Autodesk Inventor part; units mm, degrees
ref_plane "YZ Plane" through (0, 0, 0) normal (1, 0, 0) x (0, 1, 0)
ref_plane "XZ Plane" through (0, 0, 0) normal (0, 1, 0) x (-1, 0, 0)
ref_plane "XY Plane" through (0, 0, 0) normal (0, 0, 1) x (1, 0, 0)
ref_plane "Work Plane1" through (-28.594, 4.5215, 39.249) normal (0, 0, 1) x (1, 0, 0)
sketch "Sketch1" plane through (-28.594, 4.5215, 39.249) normal (0, 0, 1) x (1, 0, 0)
  circle A0 centre (23.594, 21.5215) radius 1.45
  circle A1 centre (-23.594, 21.5215) radius 1.45
  circle A2 centre (23.594, 21.5215) radius 1.45
  arc A3 (-26.094, 26.5215) -> (-28.594, 24.0215) centre (-26.094, 24.0215) ccw
  line L0 (26.094, 26.5215) -> (-26.094, 26.5215)
  arc A4 (28.594, 24.0215) -> (26.094, 26.5215) centre (26.094, 24.0215) ccw
  line L1 (28.594, 19.0215) -> (28.594, 24.0215)
  arc A5 (26.094, 16.5215) -> (28.594, 19.0215) centre (26.094, 19.0215) ccw
  line L2 (-26.094, 16.5215) -> (26.094, 16.5215)
  arc A6 (-28.594, 19.0215) -> (-26.094, 16.5215) centre (-26.094, 19.0215) ccw
  line L3 (-28.594, 24.0215) -> (-28.594, 19.0215)
  circle A7 centre (-23.594, 21.5215) radius 1.45
  point P0 (28.594, -4.5215)
extrude "Extrusion1" add sketch "Sketch1" along normal blind 7.842
sketch "Sketch2" plane through (-54.688, 31.043, 39.249) normal (0, 1, 0) x (1, 0, 0)
  line L0 (32.3438, -5.842) -> (19.8438, -5.842) construction
  line L1 (19.8438, -5.842) -> (19.8438, 0) construction
  line L2 (19.8438, 0) -> (32.3438, 0) construction
  line L3 (32.3438, 0) -> (32.3438, -5.842) construction
  line L4 (52.188, 0) -> (0, 0)
  line L5 (32.4438, 0) -> (32.4438, -6.042)
  line L6 (32.4438, -6.042) -> (19.7438, -6.042)
  line L7 (19.7438, -6.042) -> (19.7438, 0)
  point P0 (54.688, 39.249)
  dimension "d2" = 0.1
  dimension "d3" = 0.1
  dimension "d4" = 0.2
extrude "Extrusion2" cut sketch "Sketch2" against normal blind 12.908
ref_plane "Work Plane2" through (-52.188, -17, 42.6) normal (0, 0, -1) x (0, 1, 0)
sketch "Sketch3" plane through (-52.188, -17, 42.6) normal (0, 0, -1) x (0, 1, 0)
  line L0 (45.543, -5) -> (40.543, -5)
  arc A0 (38.043, -2.5) -> (40.543, -5) centre (40.543, -2.5) ccw
  line L1 (38.043, -2.5) -> (38.043, 49.688)
  arc A1 (40.543, 52.188) -> (38.043, 49.688) centre (40.543, 49.688) ccw
  line L2 (40.543, 52.188) -> (45.543, 52.188)
  arc A2 (48.043, 49.688) -> (45.543, 52.188) centre (45.543, 49.688) ccw
  line L3 (48.043, 49.688) -> (48.043, -2.5)
  arc A3 (45.543, -5) -> (48.043, -2.5) centre (45.543, -2.5) ccw
  circle A4 centre (43.043, 47.188) radius 1.45
  circle A5 centre (43.043, 0) radius 1.45
  circle A6 centre (0, 47.188) radius 3.065
  circle A7 centre (43.043, 47.188) radius 3.065
  circle A8 centre (43.043, 0) radius 3.065
  point P0 (17, 52.188)
extrude "Extrusion3" cut sketch "Sketch3" against normal blind 12.908 contours A4 | A5 | A7 | A8
properties part number "connectorHolder_V6"
Could you check a few things on this model? Use its own coordinates, in mm. A direction names the side the tool comes from. Round coordinates to 2 decimals unless told otherwise and drop trailing zeros. Write each loop counter-clockwise with the first axis right and the second up, starting at its lowest first coordinate (ties: lowest second). Pieces come first, ordered by that corner, then holes. Notation, with made-up numbers: (-20.75, -34.5) -> (33.25, -34.5) arc R21 ccw to (33.25, 1.5) -> close; hole circle Ø8 at (25.25, 43.25). An arc over 180 degrees is marked (long way). Use a Markdown table: item, result.
1. Which directions (+Z, -Z, +X, -X, +Y, -Y) give clear straight access to the entire face, cutting with the end or side of a thin tool? Please do faces 5 (the face through (-22.244, 26, 42)), 6 (the face through (-11, 26, 39.249)), 7 (the face through (-6.174, 28.874, 44.814)).
Answer key:
| item | result |
|---|---|
| face 5 | -Z, +Y, -Y |
| face 6 | -Z, +X, -X, +Y, -Y |
| face 7 | +Z |
2. If we section it at D-D (z = 46.5): List the corners of the cut face in (x, y) for me (3 decimals).
Answer key:
| item | result |
|---|---|
| outline | (-57.188, 23.543) arc R2.5 ccw to (-54.688, 21.043) -> (-2.5, 21.043) arc R2.5 ccw to (0, 23.543) -> (0, 28.543) arc R2.5 ccw to (-2.5, 31.043) -> (-54.688, 31.043) arc R2.5 ccw to (-57.188, 28.543) -> close; hole circle Ø6.13 at (-52.188, 26.043); hole circle Ø6.13 at (-5, 26.043) |
3. Please list where these lines run through material, in increasing order: probe 1 along X at (y, z) = (28, 42.5); probe 2 along X at (y, z) = (25, 46); probe 3 along Y at (x, z) = (-5, 40.95).
Answer key:
| item | result |
|---|---|
| probe 1 | x = -57.19 to -34.94, -22.24 to 0 |
| probe 2 | x = -57.19 to -55.07, -49.31 to -7.88, -2.12 to 0 |
| probe 3 | y = 21.04 to 24.59, 27.49 to 31.04 |
4. If we section it at C-C (y = 26.75): List the corners of the cut face in (x, z) for me.
Answer key:
| item | result |
|---|---|
| outline | (-57.19, 39.25) -> (-53.45, 39.25) -> (-53.45, 42.6) -> (-55.17, 42.6) -> (-55.17, 47.09) -> (-57.19, 47.09) -> close; (-50.92, 39.25) -> (-34.94, 39.25) -> (-34.94, 45.29) -> (-22.24, 45.29) -> (-22.24, 39.25) -> (-6.27, 39.25) -> (-6.27, 42.6) -> (-7.98, 42.6) -> (-7.98, 47.09) -> (-49.21, 47.09) -> (-49.21, 42.6) -> (-50.92, 42.6) -> close; (-3.73, 39.25) -> (0, 39.25) -> (0, 47.09) -> (-2.02, 47.09) -> (-2.02, 42.6) -> (-3.73, 42.6) -> close |
5. If we section it at A-A (x = -5): List the corners of the cut face in (y, z) for me, then the cut area to 3 significant figures.
Answer key:
| item | result |
|---|---|
| outline | (21.04, 39.25) -> (24.59, 39.25) -> (24.59, 42.6) -> (22.98, 42.6) -> (22.98, 47.09) -> (21.04, 47.09) -> close; (27.49, 39.25) -> (31.04, 39.25) -> (31.04, 47.09) -> (29.11, 47.09) -> (29.11, 42.6) -> (27.49, 42.6) -> close |
| area | 41.2 mm^2 |
6. For pin 1 Ø5 at (x, y) = (-26.5, 28) entering from -Z; pin 2 Ø1.8 at (x, y) = (-53, 27.5) entering from +Z; pin 3 Ø1.5 at (y, z) = (22.5, 46) entering from -X, each with a flat end and sliding along its axis, tell me the tip position at first contact or that it passes through.
Answer key:
| item | result |
|---|---|
| pin 1 | stops at z = 45.29 |
| pin 2 | stops at z = 42.6 |
| pin 3 | stops at x = -57.17 |
7. We'd pull the mould along X, two halves only. Please class faces 1 (the face through (-0.713, 21.795, 43.115)), 2 (the face through (-56.44, 21.76, 43.12)), 3 (the face through (-34.944, 26, 42)), 4 (the face through (-51.267, 28.966, 44.814)): +X half, -X half, draft (parallel to the pull), parting line (faces both ways), or undercut.
Answer key:
| item | result |
|---|---|
| face 1 | +X half |
| face 2 | -X half |
| face 3 | undercut |
| face 4 | undercut |
8. If we section it at B-B (z = 40): List the corners of the cut face in (x, y) for me, then the cut area to 3 significant figures.
Answer key:
| item | result |
|---|---|
| outline | (-57.19, 23.54) arc R2.5 ccw to (-54.69, 21.04) -> (-34.94, 21.04) -> (-34.94, 31.04) -> (-54.69, 31.04) arc R2.5 ccw to (-57.19, 28.54) -> close; (-22.24, 21.04) -> (-2.5, 21.04) arc R2.5 ccw to (0, 23.54) -> (0, 28.54) arc R2.5 ccw to (-2.5, 31.04) -> (-22.24, 31.04) -> close; hole circle Ø2.9 at (-52.19, 26.04); hole circle Ø2.9 at (-5, 26.04) |
| area | 426 mm^2 |
